Design review of the part built by this model. Coordinates are the model's own, in mm. Face numbers are marked on the shaded views. A direction names the side the tool comes from. Coordinates: 2 decimals unless noted, no trailing zeros. Write each loop counter-clockwise with the first axis right and the second up, starting at its lowest first coordinate (ties: lowest second). Pieces come first, ordered by that corner, then holes. Notation, with made-up numbers: (-7, -8.75) - (19, -8.75) arc R27 ccw to (19, 14.25) - close; hole circle Ø8 at (89.5, 83.25). An arc over 180 degrees is marked (long way). One line per item, written item: value.
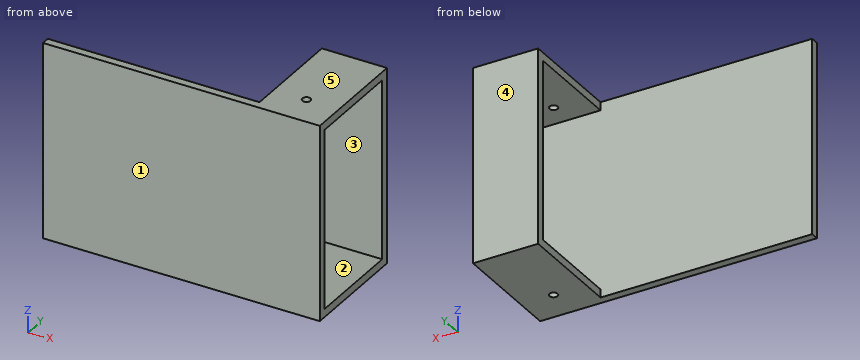
from build123d import *

# Parameters (mm, degrees)
SKETCH1_W                   = 165.1
SKETCH1_H                   = 152.4
BOSS_EXTRUDE1_DEPTH         = 6.35
SKETCH1_7_W                 = 50.8
SKETCH1_7_H                 = 152.4
BOSS_EXTRUDE2_DEPTH         = 88.9
SKETCH29_W                  = 139.7
SKETCH29_H                  = 76.2
CUT_EXTRUDE4_DEPTH          = 242.633979399
F_1_4_0_25_DIAMETER_HOLE2_D = 6.35


with BuildPart() as part:
    # Sketch1 → Boss-Extrude1 (new body)
    with BuildSketch(Plane(origin=(0, 0, 0), x_dir=(1, 0, 0), z_dir=(0, 1, 0))):
        with Locations((-133.35, 76.2)):
            Rectangle(SKETCH1_W, SKETCH1_H)
    extrude(amount=BOSS_EXTRUDE1_DEPTH)

    # Sketch1<7> → Boss-Extrude2 (add)
    with BuildSketch(Plane(origin=(0, 0, 0), x_dir=(1, 0, 0), z_dir=(0, 1, 0))):
        with Locations((-25.4, 76.2)):
            Rectangle(SKETCH1_7_W, SKETCH1_7_H)
    extrude(amount=BOSS_EXTRUDE2_DEPTH)

    # Sketch29 → Cut-Extrude4 (cut, through all)
    with BuildSketch(Plane.ZY.offset(50.8)):
        with Locations((-76.2, 44.45)):
            Rectangle(SKETCH29_W, SKETCH29_H)
    extrude(amount=-CUT_EXTRUDE4_DEPTH, mode=Mode.SUBTRACT)

    # 1/4 (0.25) Diameter Hole2 (through all)
    with Locations(Plane(origin=(0, 0, -152.4), x_dir=(-1, 0, 0), z_dir=(0, 0, -1))):
        with Locations((25.4, 25.4)):
            Hole(F_1_4_0_25_DIAMETER_HOLE2_D / 2)


solid = part.part
1. For the marked faces 1 and 2, list the 3-axis set-ups (+Z, -Z, +X, -X, +Y, -Y) from which the entire face can be reached by the end or side of a thin tool; tool diameter is ignored.
Answer block:
face 1: +Z, -Z, +X, -X, -Y
face 2: +X, -X
2. Consider section D-D, the plane x = -181. Write out the cut boundary in (y, z), then the cut area to 3 significant figures.
Answer block:
outline: (0, -152.4) - (6.35, -152.4) - (6.35, 0) - (0, 0) - close
area: 968 mm^2
3. Insertion check: pin 1 Ø3 at (x, z) = (-186, -73) entering from +Y; pin 2 Ø1.5 at (x, z) = (-72, -82.5) entering from +Y; pin 3 Ø6 at (y, z) = (77.5, -65) entering from -X. Each pin has a flat end and moves straight along its axis. Give the tip position at first contact, or say it passes through.
Answer block:
pin 1: stops at y = 6.35
pin 2: stops at y = 6.35
pin 3: passes through
4. Mouldability with a two-part tool opening along Z and no side actions: class the marked faces 3, 4 and 5 as released by +Z, released by -Z, zero draft, split by the parting line, or undercut.
Answer block:
face 3: undercut
face 4: zero draft
face 5: released by +Z
5. Consider section C-C, the plane y = 17.5. Write out the cut boundary in (x, z).
Answer block:
outline: (-50.8, -152.4) - (0, -152.4) - (0, -146.05) - (-50.8, -146.05) - close; (-50.8, -6.35) - (0, -6.35) - (0, 0) - (-50.8, 0) - close
6. Wall thickness on line 1 along Y through (x, z) = (-25.4, -2.5) (3 decimals); line 2 along Y through (x, z) = (-25, -150); line 3 along Y through (x, z) = (-124, -40): over which ranges is each line inside the solid? List them lowest first.
Answer block:
line 1: y = 0 to 22.225, 28.575 to 88.9
line 2: y = 0 to 22.25, 28.55 to 88.9
line 3: y = 0 to 6.35
7. Consider section B-B, the plane x = -25.4. Write out the cut boundary in (y, z) (3 decimals), then the cut area to 3 significant figures.
Answer block:
outline: (0, -152.4) - (22.225, -152.4) - (22.225, -146.05) - (6.35, -146.05) - (6.35, -6.35) - (22.225, -6.35) - (22.225, 0) - (0, 0) - close; (28.575, -152.4) - (88.9, -152.4) - (88.9, 0) - (28.575, 0) - (28.575, -6.35) - (82.55, -6.35) - (82.55, -146.05) - (28.575, -146.05) - close
area: 2,820 mm^2
8. Consider section A-A, the plane z = -90. Write out the cut boundary in (x, y).
Answer block:
outline: (-215.9, 0) - (0, 0) - (0, 6.35) - (-215.9, 6.35) - close; (-50.8, 82.55) - (0, 82.55) - (0, 88.9) - (-50.8, 88.9) - close
